The listing builds one solid part. Answer for the finished solid, in the listing's coordinates (mm). Face numbers are marked on the shaded views. Round coordinates to 2 decimals unless told otherwise and drop trailing zeros. Loops run counter-clockwise (first coordinate to the right, second up) from the corner with the lowest first, then second, coordinate; pieces in that order, holes last. Notation, with made-up numbers: M 69.25,6 L 101.25,6 A17 ccw 101.25,29 Z; hole C 74,25.5 d5. An arc over 180 degrees is marked long. Put each result on its own line as item: value. Start each with the question number.
(1) Section D-D, the plane x = 20 is taken. Determine the outline of the cut face in (y, z).
(2) Section C-C, the plane y = 0 is taken. Determine the outline of the cut face in (x, z), then the cut area to 3 significant figures.
(3) Determine the mould class of the marked faces 1, 2 and 3 for opening direction Z: released by +Z, released by -Z, zero draft, split by the parting line, or undercut.
(4) Section B-B, the plane z = 4 is taken. Determine the outline of the cut face in (x, y).
(5) Section A-A, the plane x = -3 is taken. Determine the outline of the cut face in (y, z), then the cut area to 3 significant figures.
(6) Straight lines are drawn through the part: line 1 (X direction, y = 3.5, z = 6.25); line 2 (Y direction, x = -35, z = 3.5); line 3 (X direction, y = -0.25, z = 4). For each, find the intervals that lie inside material, in ascending order.
```python
from build123d import *

# Parameters (mm, degrees)
F0_W     = 80
F0_H     = 12.6
F1_DEPTH = 12.5
F3_DEPTH = 12.6
F4_D     = 3.3


with BuildPart() as f1:
    # F0 (on Top) → F1 (new body)
    with BuildSketch(Plane.XY):
        Rectangle(F0_W, F0_H)
    extrude(amount=F1_DEPTH)

    # F2 (on face) → F3 (cut, through all)
    with BuildSketch(Plane.XZ.offset(6.3)):
        with BuildLine():
            ThreePointArc((0, 3.2396013553), (4.6298006013, 2.324920383), (7.25, 6.25))
            ThreePointArc((7.25, 6.25), (4.6298006013, 10.175079617), (0, 9.2603986447))
            ThreePointArc((0, 9.2603986447), (0.925079617, 7.8798006013), (1.25, 6.25))
            ThreePointArc((1.25, 6.25), (0.925079617, 4.6201993987), (0, 3.2396013553))
        make_face()
        with BuildLine():
            ThreePointArc((1.25, 6.25), (0.925079617, 7.8798006013), (0, 9.2603986447))
            ThreePointArc((0, 9.2603986447), (-1.25, 6.25), (0, 3.2396013553))
            ThreePointArc((0, 3.2396013553), (0.925079617, 4.6201993987), (1.25, 6.25))
        make_face()
        with BuildLine():
            ThreePointArc((0, 3.2396013553), (-1.25, 6.25), (0, 9.2603986447))
            ThreePointArc((0, 9.2603986447), (-7.25, 6.25), (0, 3.2396013553))
        make_face()
    extrude(amount=-F3_DEPTH, mode=Mode.SUBTRACT)

    # F4 (through all)
    with Locations(Plane(origin=(0, 0, 0), x_dir=(1, 0, 0), z_dir=(0, 0, -1))):
        with Locations((-20, 0), (-35, 0), (20, 0), (35, 0)):
            Hole(F4_D / 2)


solid = f1.part
```
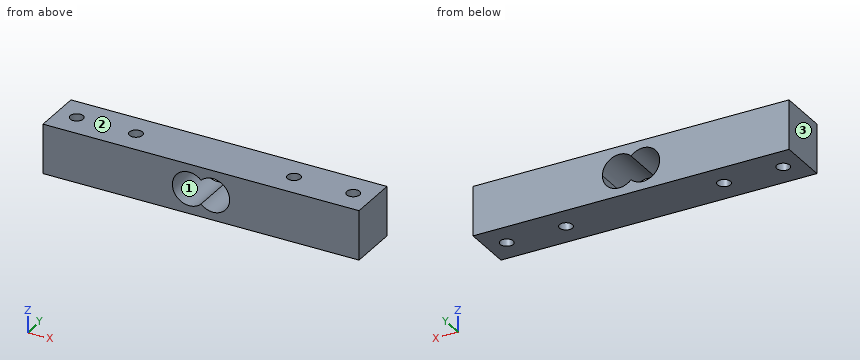
Recorded:
1. outline: M -6.3,0 L -1.65,0 L -1.65,12.5 L -6.3,12.5 Z; M 1.65,0 L 6.3,0 L 6.3,12.5 L 1.65,12.5 Z
2. outline: M -40,0 L -36.65,0 L -36.65,12.5 L -40,12.5 Z; M -33.35,0 L -21.65,0 L -21.65,12.5 L -33.35,12.5 Z; M -18.35,0 L 18.35,0 L 18.35,12.5 L -18.35,12.5 Z; M 21.65,0 L 33.35,0 L 33.35,12.5 L 21.65,12.5 Z; M 36.65,0 L 40,0 L 40,12.5 L 36.65,12.5 Z; hole M 0,3.24 A4.25 ccw long 0,9.26 A4.25 ccw long Z
2. area: 732 mm²
3. face 1: undercut
3. face 2: released by +Z
3. face 3: zero draft
4. outline: M -40,-6.3 L -6.61,-6.3 L -6.61,6.3 L -40,6.3 Z; M 6.61,-6.3 L 40,-6.3 L 40,6.3 L 6.61,6.3 Z; hole C -35,0 d3.3; hole C -20,0 d3.3; hole C 20,0 d3.3; hole C 35,0 d3.3
5. outline: M -6.3,0 L 6.3,0 L 6.3,2 L -6.3,2 Z; M -6.3,10.5 L 6.3,10.5 L 6.3,12.5 L -6.3,12.5 Z
5. area: 50.4 mm²
6. line 1: x = -40 to -7.25, 7.25 to 40
6. line 2: y = -6.3 to -1.65, 1.65 to 6.3
6. line 3: x = -40 to -36.63, -33.37 to -21.63, -18.37 to -6.61, 6.61 to 18.37, 21.63 to 33.37, 36.63 to 40
